Could you check a few things on this model? Use its own coordinates, in mm. Give positions to 0.01 mm unless a question says otherwise; leave off trailing zeros. Write each loop counter-clockwise with the first axis right and the second up, starting at its lowest first coordinate (ties: lowest second). Pieces come first, ordered by that corner, then holes. Notation, with made-up numbers: (49, 38) - (80, 38) arc R11 ccw to (80, 44) - close; hole circle Ø1 at (8, -40). An arc over 180 degrees is marked (long way). Answer in a Markdown table with one row per item.
from build123d import *

# Parameters (mm, degrees)
BOSS_EXTRUDE1_DEPTH = 7
SKETCH2_R           = 2.2
CUT_EXTRUDE1_DEPTH  = 4


with BuildPart() as part:
    # Sketch1 → Boss-Extrude1 (new body)
    with BuildSketch(Plane(origin=(0, 0, 0), x_dir=(1, 0, 0), z_dir=(0, 1, 0))):
        with BuildLine():
            Line((0, 0), (-17.05, 0))
            Line((-17.05, 0), (-17.05, 4))
            Line((-17.05, 4), (-15.05, 4))
            ThreePointArc((-15.05, 4), (-12.5, 1.45), (-9.95, 4))
            Line((-9.95, 4), (0, 4))
            Line((0, 4), (0, 0))
        make_face()
    extrude(amount=BOSS_EXTRUDE1_DEPTH)

    # Sketch2 → Cut-Extrude1 (cut)
    with BuildSketch(Plane.XY):
        with Locations((-5, 3.5)):
            Circle(SKETCH2_R)
    extrude(amount=-CUT_EXTRUDE1_DEPTH, mode=Mode.SUBTRACT)

    # Mirror1: part across plane


with BuildPart() as part_1:
    add(part.part)
    add(part.part.mirror(Plane(origin=(0, 0, 0), x_dir=(0, 0, 1), z_dir=(1, 0, 0))))


solid = part_1.part
1) Will this pin go through, and if not, where does the flat tip stop? P1, Ø1, axis at x = -5.5, y = 4, coming from the -Z side.
Check values:
| item | result |
|---|---|
| P1 | passes through |
2) Imagine slicing it at B-B (z = -2.75). List the corners of the cut face in (x, y) for me.
Check values:
| item | result |
|---|---|
| outline | (-17.05, 0) - (-14.72, 0) - (-14.72, 7) - (-17.05, 7) - close; (-10.28, 0) - (10.28, 0) - (10.28, 7) - (-10.28, 7) - close; (14.72, 0) - (17.05, 0) - (17.05, 7) - (14.72, 7) - close; hole circle Ø4.4 at (-5, 3.5); hole circle Ø4.4 at (5, 3.5) |
3) Imagine slicing it at A-A (y = 3.5). List the corners of the cut face in (x, z) for me, then the cut area to 3 significant figures.
Check values:
| item | result |
|---|---|
| outline | (-17.05, -4) - (-15.05, -4) arc R2.55 cw to (-9.95, -4) - (-7.2, -4) - (-7.2, 0) - (-17.05, 0) - close; (-2.8, -4) - (2.8, -4) - (2.8, 0) - (-2.8, 0) - close; (7.2, -4) - (9.95, -4) arc R2.55 cw to (15.05, -4) - (17.05, -4) - (17.05, 0) - (7.2, 0) - close |
| area | 80.8 mm2 |
4) If I drill on line 1 (X direction, y = 0.75, z = -1.95); line 2 (X direction, y = 0.5, z = -1.65); line 3 (X direction, y = 3.25, z = -2.6), over which ranges is the centre line in solid material (lowest first)?
Check values:
| item | result |
|---|---|
| line 1 | x = -17.05 to -14.02, -10.98 to 10.98, 14.02 to 17.05 |
| line 2 | x = -17.05 to -13.49, -11.51 to 11.51, 13.49 to 17.05 |
| line 3 | x = -17.05 to -14.63, -10.37 to -7.19, -2.81 to 2.81, 7.19 to 10.37, 14.63 to 17.05 |
5) Imagine slicing it at D-D (x = -12.5). List the corners of the cut face in (y, z) for me, then the cut area to 4 significant figures.
Check values:
| item | result |
|---|---|
| outline | (0, -1.45) - (7, -1.45) - (7, 0) - (0, 0) - close |
| area | 10.15 mm2 |
6) We'd pull the mould along X, two halves only. Please class faces 1 (the face through (16, 3, -4)), 2 (the face through (-17.05, 3, -2)), 3 (the face through (17.05, 3, -2)), 4 (the face through (2.968, 2.657, -1.972)): +X half, -X half, draft (parallel to the pull), parting line (faces both ways), or undercut.
Check values:
| item | result |
|---|---|
| face 1 | draft |
| face 2 | -X half |
| face 3 | +X half |
| face 4 | undercut |
7) Imagine slicing it at C-C (x = -5). List the corners of the cut face in (y, z) for me.
Check values:
| item | result |
|---|---|
| outline | (0, -4) - (1.3, -4) - (1.3, 0) - (0, 0) - close; (5.7, -4) - (7, -4) - (7, 0) - (5.7, 0) - close |
